Geometry check sheet. Reference: the model listing, model coordinates, mm. Face numbers are marked on the shaded views. A direction names the side the tool comes from. Coordinates: 2 decimals unless noted, no trailing zeros. Write each loop counter-clockwise with the first axis right and the second up, starting at its lowest first coordinate (ties: lowest second). Pieces come first, ordered by that corner, then holes. Notation, with made-up numbers: (79, 24.5) - (117, 24.5) arc R11 ccw to (117, 32.5) - close; hole circle Ø1 at (33.5, 4). An arc over 180 degrees is marked (long way). Answer as a JSON object with one key per item and string values. Group by question number.
Autodesk Inventor part; units mm, degrees
ref_plane "YZ Plane" through (0, 0, 0) normal (1, 0, 0) x (0, 1, 0)
ref_plane "XZ Plane" through (0, 0, 0) normal (0, 1, 0) x (-1, 0, 0)
ref_plane "XY Plane" through (0, 0, 0) normal (0, 0, 1) x (1, 0, 0)
sketch "Sketch1" plane through (0, 0, 0) normal (0, 0, 1) x (1, 0, 0)
  line L0 (0, 0) -> (50.8, 0)
  line L1 (50.8, 0) -> (50.8, 101.6)
  line L2 (50.8, 101.6) -> (0, 101.6)
  line L3 (0, 101.6) -> (0, 0)
  dimension "d3" = 50.8
  dimension "d4" = 101.6
extrude "Extrusion1" add sketch "Sketch1" along normal blind 25.4
shell "Shell1" thickness 3.175 removed faces 2 at (33.8667, 101.6, 16.9333) at (16.9333, 0, 16.9333)
sketch "Sketch2" plane through (0, 0, 0) normal (0, 0, -1) x (-1, 0, 0)
  line L0 (-50.8, 101.6) -> (0, 101.6)
  line L1 (-50.8, 0) -> (-50.8, 101.6)
  line L2 (-50.8, 50.8) -> (-50.8, 101.6)
  line L3 (-50.8, 101.6) -> (0, 101.6)
  line L4 (0, 101.6) -> (-50.8, 50.8)
  dimension "d5" = 50.8
extrude "Extrusion2" cut sketch "Sketch2" against normal through all
sketch "Sketch3" plane through (0, 0, 0) normal (-1, 0, 0) x (0, 0, 1)
  line L0 (0, 101.6) -> (25.4, 101.6)
  line L1 (0, 101.6) -> (0, 0)
  arc A0 (6.35, 76.2) -> (19.05, 76.2) centre (12.7, 76.2) ccw
  line L2 (6.35, 76.2) -> (6.35, 101.6)
  line L3 (19.05, 76.2) -> (19.05, 101.6)
  dimension "d8" = 25.4
  dimension "d9" = 6.35
  dimension "d10" = 12.7
extrude "Extrusion3" cut sketch "Sketch3" against normal through all
chamfer "Chamfer1" distance 3.175 angle 45 2 edges at (1.5875, 100.0125, 6.35) (1.5875, 100.0125, 19.05)
sketch "Sketch4" plane through (0, 0, 25.4) normal (0, 0, 1) x (1, 0, 0)
  line L0 (50.8, 50.8) -> (0, 101.6)
  line L1 (0, 0) -> (0, 101.6)
  line L2 (0, 101.6) -> (0, 95.25)
  line L3 (6.35, 95.25) -> (0, 101.6)
  line L4 (0, 95.25) -> (6.35, 95.25)
  dimension "d16" = 6.35
extrude "Extrusion4" cut sketch "Sketch4" against normal through all
properties part number "FrameSideBumperMounts" material "Aluminum-6061"
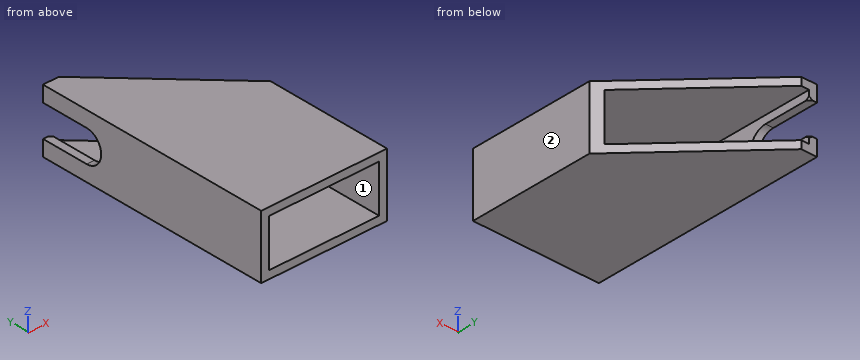
(1) Material ranges on L1, parallel to Z at x = 14, y = 80.5 (3 decimals); L2, parallel to X at y = 14, z = 6.75 (3 decimals); L3, parallel to X at y = 53, z = 9.25 (3 decimals), recorded low to high. Write a range as [from, to].
(2) Set-up check for the marked faces 1 and 2: record each of +Z, -Z, +X, -X, +Y, -Y from which the full face is reachable in a straight line by a thin tool's end or side.
(3) Section check C-C (y = 88). Record the cut outline in (x, z) (3 decimals), and give its area (3 significant figures).
(4) Section check B-B (z = 12.7). Record the cut outline in (x, y) (3 decimals), and give its area (3 significant figures).
(5) Section check D-D (y = 12). Record the cut outline in (x, z) (3 decimals), and give its area (3 significant figures).
(6) Gauge pin test, flat ends, axial feed: pin 1 (4 mm diameter, centred on y = 62.5, z = 20, fed in from +X) (3 decimals); pin 2 (2.5 mm diameter, centred on x = 2, y = 84.5, fed in from -Z); pin 3 (4 mm diameter, centred on x = 41.5, z = 5, fed in from +Y). Record the tip position at first contact, or that the pin passes through.
(7) Section check A-A (x = 36). Record the cut outline in (y, z) (3 decimals).
Conclusion:
{
 "1": {"L1": "z = [0, 3.175], [22.225, 25.4]", "L2": "x = [0, 3.175], [47.625, 50.8]", "L3": "x = [0, 3.175], [47.625, 48.6]"},
 "2": {"face 1": "+Y, -Y", "face 2": "+Z, -Z, +X, +Y, -Y"},
 "3": {"outline": "(0, 0) - (13.6, 0) - (13.6, 3.175) - (3.175, 3.175) - (3.175, 6.35) - (0, 6.35) - close; (0, 19.05) - (3.175, 19.05) - (3.175, 22.225) - (13.6, 22.225) - (13.6, 25.4) - (0, 25.4) - close", "area": "107 mm^2"},
 "4": {"outline": "(0, 0) - (3.175, 0) - (3.175, 69.85) - (0, 69.85) - close; (47.625, 0) - (50.8, 0) - (50.8, 50.8) - (47.625, 53.975) - close", "area": "388 mm^2"},
 "5": {"outline": "(0, 0) - (50.8, 0) - (50.8, 25.4) - (0, 25.4) - close; hole (3.175, 3.175) - (47.625, 3.175) - (47.625, 22.225) - (3.175, 22.225) - close", "area": "444 mm^2"},
 "6": {"pin 1": "stops at x = 3.175", "pin 2": "stops at z = 0", "pin 3": "stops at y = 60.92"},
 "7": {"outline": "(0, 0) - (65.6, 0) - (65.6, 3.175) - (0, 3.175) - close; (0, 22.225) - (65.6, 22.225) - (65.6, 25.4) - (0, 25.4) - close"}
}
